Could you check a few things on this model? Use its own coordinates, in mm. Give positions to 0.01 mm unless a question says otherwise; leave off trailing zeros. Loops run counter-clockwise (first coordinate to the right, second up) from the corner with the lowest first, then second, coordinate; pieces in that order, holes last. Notation, with made-up numbers: (55, 33.25) - (87, 33.25) arc R29 cw to (87, 67.25) - close; hole circle Ø9 at (4.25, 40). An arc over 180 degrees is marked (long way). Use CSV: the item, a comma, the result in double quotes.
from build123d import *

# Parameters (mm, degrees)
SKETCH1_W               = 306
SKETCH1_H               = 396
BOSS_EXTRUDE1_DEPTH     = 1
SKETCH2_R               = 1.5
CUT_EXTRUDE1_DEPTH      = 251.227896127
SKETCH3_R               = 8
CUT_EXTRUDE2_DEPTH      = 251.227896127
SKETCH4_R               = 1.5
SKETCH4_W               = 80
SKETCH4_H               = 80
CUT_EXTRUDE3_DEPTH      = 251.227896127
SKETCH6_R               = 1.5
CUT_EXTRUDE4_DEPTH      = 251.227896127
MIRROR4_COPY_1_SKETCH_R = 1.5
MIRROR4_COPY_1_DEPTH    = 251.227896127
SKETCH8_R               = 1.5
SKETCH8_W               = 100
SKETCH8_H               = 35
CUT_EXTRUDE6_DEPTH      = 251.227896127


with BuildPart() as part:
    # Sketch1 → Boss-Extrude1 (new body)
    with BuildSketch(Plane(origin=(0, 0, 0), x_dir=(1, 0, 0), z_dir=(0, 1, 0))):
        Rectangle(SKETCH1_W, SKETCH1_H)
    extrude(amount=BOSS_EXTRUDE1_DEPTH)

    # Sketch2 → Cut-Extrude1 (cut, through all)
    with BuildSketch(Plane(origin=(0, 1, 0), x_dir=(1, 0, 0), z_dir=(0, 1, 0))):
        with Locations(Location((0, -18.5, 0), (0, 0, 270))):
            Circle(SKETCH2_R)
        with Locations(Location((0, -138.5, 0), (0, 0, 270))):
            Circle(SKETCH2_R)
        with BuildLine():
            Line((1.5, -23.5), (1.5, -133.5))
            ThreePointArc((1.5, -133.5), (0, -135), (-1.5, -133.5))
            Line((-1.5, -133.5), (-1.5, -23.5))
            ThreePointArc((-1.5, -23.5), (0, -22), (1.5, -23.5))
        make_face()
    extrude(amount=-CUT_EXTRUDE1_DEPTH, mode=Mode.SUBTRACT)

    # Sketch3 → Cut-Extrude2 (cut, through all)
    with BuildSketch(Plane(origin=(0, 1, 0), x_dir=(1, 0, 0), z_dir=(0, 1, 0))):
        with Locations(Location((-50, 20, 0), (0, 0, 270))):
            Circle(SKETCH3_R)
    cut_extrude2 = extrude(amount=-CUT_EXTRUDE2_DEPTH, mode=Mode.SUBTRACT)

    # Mirror1: Cut-Extrude2 across plane
    add(cut_extrude2.mirror(Plane(origin=(0, 0, 0), x_dir=(0, 0, 1), z_dir=(1, 0, 0))), mode=Mode.SUBTRACT)

    # Sketch4 → Cut-Extrude3 (cut, through all)
    with BuildSketch(Plane(origin=(0, 1, 0), x_dir=(1, 0, 0), z_dir=(0, 1, 0))):
        with Locations(Location((-96, 140, 0), (0, 0, 270))):
            Circle(SKETCH4_R)
        with Locations(Location((-6, 140, 0), (0, 0, 270))):
            Circle(SKETCH4_R)
        with Locations(Location((-96, 50, 0), (0, 0, 270))):
            Circle(SKETCH4_R)
        with Locations(Location((-6, 50, 0), (0, 0, 270))):
            Circle(SKETCH4_R)
        with Locations((-51, 95)):
            Rectangle(SKETCH4_W, SKETCH4_H)
    cut_extrude3 = extrude(amount=-CUT_EXTRUDE3_DEPTH, mode=Mode.SUBTRACT)

    # Mirror2: Cut-Extrude3 across plane
    add(cut_extrude3.mirror(Plane(origin=(0, 0, 0), x_dir=(0, 0, 1), z_dir=(1, 0, 0))), mode=Mode.SUBTRACT)

    # Sketch6 → Cut-Extrude4 (cut, through all)
    with BuildSketch(Plane(origin=(0, 1, 0), x_dir=(1, 0, 0), z_dir=(0, 1, 0))):
        with Locations(Location((-143, 91, 0), (0, 0, 270))):
            Circle(SKETCH6_R)
        with BuildLine():
            Line((-153, 148), (-103, 148))
            ThreePointArc((-103, 148), (-102.5, 147.5), (-103, 147))
            Line((-103, 147), (-153, 147))
            ThreePointArc((-153, 147), (-153.5, 147.5), (-153, 148))
        make_face()
    cut_extrude4 = extrude(amount=-CUT_EXTRUDE4_DEPTH, mode=Mode.SUBTRACT)

    # Mirror3: Cut-Extrude4 across plane
    add(cut_extrude4.mirror(Plane.XY), mode=Mode.SUBTRACT)

    # Mirror4: Cut-Extrude4 across plane
    add(cut_extrude4.mirror(Plane(origin=(0, 0, 0), x_dir=(0, 0, 1), z_dir=(1, 0, 0))), mode=Mode.SUBTRACT)

    # Mirror4 copy 1 sketch → Mirror4 copy 1 (cut, through all)
    with BuildSketch(Plane(origin=(0, 1, 0), x_dir=(-1, 0, 0), z_dir=(0, 1, 0))):
        with Locations(Location((-143, 91, 0), (0, 0, 270))):
            Circle(MIRROR4_COPY_1_SKETCH_R)
        with BuildLine():
            Line((-153, 148), (-103, 148))
            ThreePointArc((-103, 148), (-102.5, 147.5), (-103, 147))
            Line((-103, 147), (-153, 147))
            ThreePointArc((-153, 147), (-153.5, 147.5), (-153, 148))
        make_face()
    extrude(amount=-MIRROR4_COPY_1_DEPTH, mode=Mode.SUBTRACT)

    # Sketch8 → Cut-Extrude6 (cut, through all)
    with BuildSketch(Plane(origin=(0, 1, 0), x_dir=(1, 0, 0), z_dir=(0, 1, 0))):
        with Locations(Location((-55, 185.5, 0), (0, 0, 270))):
            Circle(SKETCH8_R)
        with Locations(Location((-55, 160.5, 0), (0, 0, 270))):
            Circle(SKETCH8_R)
        with Locations(Location((55, 160.5, 0), (0, 0, 90))):
            Circle(SKETCH8_R)
        with Locations(Location((55, 185.5, 0), (0, 0, 90))):
            Circle(SKETCH8_R)
        with Locations((0, 173)):
            Rectangle(SKETCH8_W, SKETCH8_H)
    extrude(amount=-CUT_EXTRUDE6_DEPTH, mode=Mode.SUBTRACT)


solid = part.part
1) I'm going to push a flat-ended pin straight in: P1, Ø2.5, axis at x = 0, z = 138.5, coming from the -Y side. Where does the tip first touch, or does it pass through?
Answer below:
P1,"passes through"
2) Suppose I cut it at C-C (x = -27). Please give me the cut outline in (y, z).
Answer below:
outline,"(0, -198) - (1, -198) - (1, -190.5) - (0, -190.5) - close; (0, -155.5) - (1, -155.5) - (1, -135) - (0, -135) - close; (0, -55) - (1, -55) - (1, 198) - (0, 198) - close"
3) I need wall thicknesses on line 1 along Z through (x, y) = (-109, 0.8); line 2 along X through (y, z) = (0.55, -91); line 3 along X through (y, z) = (0.2, -50). Which ranges of each line are inside material? Lowest first, please.
Answer below:
line 1,"z = -198 to -148, -147 to 147, 148 to 198"
line 2,"x = -153 to -144.5, -141.5 to -91, -11 to 11, 91 to 141.5, 144.5 to 153"
line 3,"x = -153 to -97.5, -94.5 to -7.5, -4.5 to 4.5, 7.5 to 94.5, 97.5 to 153"
4) We'd pull the mould along Z, two halves only. Please class faces 1 (the cylindrical face through (-42.068, 0.507, -21.041)), 2 (the flat face through (-2, 1, -3)): +Z half, -Z half, draft (parallel to the pull), parting line (faces both ways), or undercut.
Answer below:
face 1,"undercut"
face 2,"draft"
5) Suppose I cut it at D-D (y = 0.2). State how many separate pieces and enclosed holes the cut face has, plus the area to 3 significant figures.
Answer below:
separate pieces,"1"
enclosed holes,"24"
area,"104,000 mm2"
6) Suppose I cut it at B-B (z = -118.5). Please give me the cut outline in (x, y).
Answer below:
outline,"(-153, 0) - (-91, 0) - (-91, 1) - (-153, 1) - close; (-11, 0) - (11, 0) - (11, 1) - (-11, 1) - close; (91, 0) - (153, 0) - (153, 1) - (91, 1) - close"
7) Suppose I cut it at A-A (x = 70). Please give me the cut outline in (y, z), plus the area to 3 significant figures.
Answer below:
outline,"(0, -198) - (1, -198) - (1, -135) - (0, -135) - close; (0, -55) - (1, -55) - (1, 198) - (0, 198) - close"
area,"316 mm2"
